Build history of the part. All positions in model axes, mm. A direction names the side the tool comes from. Give positions to 0.01 mm unless a question says otherwise; leave off trailing zeros. Loops run counter-clockwise (first coordinate to the right, second up) from the corner with the lowest first, then second, coordinate; pieces in that order, holes last. Notation, with made-up numbers: M 64,-6 L 122,-6 A29 ccw 122,22 Z; hole C -26,81.5 d2. An arc over 180 degrees is marked long. Answer in a Markdown table with one row per item. Add a question column.
```python
from build123d import *

# Parameters (mm, degrees)
SKETCH9_W           = 299
SKETCH9_H           = 464
SKETCH9_R           = 12.5
SKETCH9_R_2         = 10.287
SKETCH9_W_2         = 187.325
SKETCH9_H_2         = 265.1125
BOSS_EXTRUDE7_DEPTH = 3.175
FILLET4_R           = 10
FILLET5_R           = 12.7
SKETCH10_R          = 3
CUT_EXTRUDE1_DEPTH  = 3.175


with BuildPart() as part:
    # Sketch9 → Boss-Extrude7 (new body)
    with BuildSketch(Plane(origin=(0, 0, 0), x_dir=(1, 0, 0), z_dir=(0, 1, 0))):
        with Locations((0, 232)):
            Rectangle(SKETCH9_W, SKETCH9_H)
        with Locations(Location((-98.7, 63.5, 0), (0, 0, 270))):
            Circle(SKETCH9_R, mode=Mode.SUBTRACT)
        with Locations(Location((111.4, 76.2, 0), (0, 0, 270))):
            Circle(SKETCH9_R_2, mode=Mode.SUBTRACT)
        with Locations(Location((111.4, 38.1, 0), (0, 0, 270))):
            Circle(SKETCH9_R_2, mode=Mode.SUBTRACT)
        with Locations(Location((73.3, 76.2, 0), (0, 0, 270))):
            Circle(SKETCH9_R_2, mode=Mode.SUBTRACT)
        with Locations(Location((73.3, 38.1, 0), (0, 0, 270))):
            Circle(SKETCH9_R_2, mode=Mode.SUBTRACT)
        with Locations((9.5, 252)):
            Rectangle(SKETCH9_W_2, SKETCH9_H_2, mode=Mode.SUBTRACT)
        with BuildLine():
            Line((6.870225615, 415.1), (-6.870225615, 415.1))
            ThreePointArc((-6.870225615, 415.1), (0, 438.7), (6.870225615, 415.1))
        make_face(mode=Mode.SUBTRACT)
    extrude(amount=BOSS_EXTRUDE7_DEPTH)

    # Fillet4
    fillet4_edges = [part.edges().sort_by_distance(p)[0] for p in [
        (-149.5, 1.5875, -464),
        (149.5, 1.5875, -464),
        (149.5, 1.5875, 0),
        (-149.5, 1.5875, 0),
    ]]
    fillet(fillet4_edges, radius=FILLET4_R)

    # Fillet5
    fillet5_edges = [part.edges().sort_by_distance(p)[0] for p in [
        (103.1625, 1.5875, -119.44375),
        (103.1625, 1.5875, -384.55625),
        (-84.1625, 1.5875, -384.55625),
        (-84.1625, 1.5875, -119.44375),
    ]]
    fillet(fillet5_edges, radius=FILLET5_R)

    # Sketch10 → Cut-Extrude1 (cut)
    with BuildSketch(Plane(origin=(0, 3.175, 0), x_dir=(1, 0, 0), z_dir=(0, 1, 0))):
        with Locations(Location((-138.5, 11, 0), (0, 0, 270))):
            Circle(SKETCH10_R)
        with Locations(Location((-46.166666667, 11, 0), (0, 0, 270))):
            Circle(SKETCH10_R)
        with Locations(Location((46.166666667, 11, 0), (0, 0, 270))):
            Circle(SKETCH10_R)
        with Locations(Location((138.5, 11, 0), (0, 0, 270))):
            Circle(SKETCH10_R)
        with Locations(Location((-138.5, 84.666666667, 0), (0, 0, 270))):
            Circle(SKETCH10_R)
        with Locations(Location((-138.5, 158.333333333, 0), (0, 0, 270))):
            Circle(SKETCH10_R)
        with Locations(Location((-138.5, 232, 0), (0, 0, 270))):
            Circle(SKETCH10_R)
        with Locations(Location((-138.5, 305.666666667, 0), (0, 0, 270))):
            Circle(SKETCH10_R)
        with Locations(Location((-138.5, 379.333333333, 0), (0, 0, 270))):
            Circle(SKETCH10_R)
        with Locations(Location((-138.5, 453, 0), (0, 0, 270))):
            Circle(SKETCH10_R)
        with Locations(Location((138.5, 84.666666667, 0), (0, 0, 270))):
            Circle(SKETCH10_R)
        with Locations(Location((138.5, 158.333333333, 0), (0, 0, 270))):
            Circle(SKETCH10_R)
        with Locations(Location((138.5, 232, 0), (0, 0, 270))):
            Circle(SKETCH10_R)
        with Locations(Location((138.5, 305.666666667, 0), (0, 0, 270))):
            Circle(SKETCH10_R)
        with Locations(Location((138.5, 379.333333333, 0), (0, 0, 270))):
            Circle(SKETCH10_R)
        with Locations(Location((-46.166666667, 453, 0), (0, 0, 270))):
            Circle(SKETCH10_R)
        with Locations(Location((46.166666667, 453, 0), (0, 0, 270))):
            Circle(SKETCH10_R)
        with Locations(Location((138.5, 453, 0), (0, 0, 270))):
            Circle(SKETCH10_R)
    extrude(amount=-CUT_EXTRUDE1_DEPTH, mode=Mode.SUBTRACT)


solid = part.part
```
(1) Slice it at B-B, the plane z = -364.5. Give the cut face in (x, y) (1 decimal), then the cut area to 3 significant figures.
(2) Slice it at A-A, the plane x = -20. Give the cut face in (y, z) (3 decimals), then the cut area to 3 significant figures.
(3) Pin check, flat tip, straight feed: pin 1 (5.5 mm diameter, centred on x = 138.5, z = -84.67, fed in from +Y). Stop position of the tip, or through.
(4) Slice it at D-D, the plane x = 67.5. Give the cut face in (y, z) (3 decimals), then the cut area to 3 significant figures.
(5) Tool access for faces 1 (the cylindrical face through (-146.65, 1.61, -3.01)), 2 (the cylindrical face through (99.54, 1.61, -380.74)): list every direction of +Z, -Z, +X, -X, +Y, -Y with a clear straight run to the whole face (end or side of a thin tool).
(6) Slice it at C-C, the plane z = -38.1. Give the cut face in (x, y) (3 decimals).
(7) Pull direction Z, two halves, no side cores. Call faces 3 (the cylindrical face through (146.49, 1.61, -2.85)), 4 (the cylindrical face through (-146.65, 1.61, -460.99)), 5 (the cylindrical face through (-80.343, 1.61, -123.065)), 6 (the flat face through (-102, 0, -235)): +Z half, -Z half, draft (parallel to the pull), parting line (faces both ways), or undercut.
(8) Wall check: line 1 (X direction, y = 1.95, z = -453); line 2 (X direction, y = 2.25, z = -237); line 3 (Z direction, x = -10, y = 0.5). Give the ranges that are in metal, low to high.
Solution:
| question | item | result |
|---|---|---|
| 1 | outline | M -149.5,0 L -84.2,0 L -84.2,3.2 L -149.5,3.2 Z; M 103.2,0 L 149.5,0 L 149.5,3.2 L 103.2,3.2 Z |
| 1 | area | 355 mm^2 |
| 2 | outline | M 0,-464 L 3.175,-464 L 3.175,-384.556 L 0,-384.556 Z; M 0,-119.444 L 3.175,-119.444 L 3.175,0 L 0,0 Z |
| 2 | area | 631 mm^2 |
| 3 | pin 1 | through |
| 4 | outline | M 0,-464 L 3.175,-464 L 3.175,-384.556 L 0,-384.556 Z; M 0,-119.444 L 3.175,-119.444 L 3.175,-84.696 L 0,-84.696 Z; M 0,-67.704 L 3.175,-67.704 L 3.175,-46.596 L 0,-46.596 Z; M 0,-29.604 L 3.175,-29.604 L 3.175,0 L 0,0 Z |
| 4 | area | 524 mm^2 |
| 5 | face 1 | +Z, -X, +Y, -Y |
| 5 | face 2 | +Y, -Y |
| 6 | outline | M -149.5,0 L 63.013,0 L 63.013,3.175 L -149.5,3.175 Z; M 83.587,0 L 101.113,0 L 101.113,3.175 L 83.587,3.175 Z; M 121.687,0 L 149.5,0 L 149.5,3.175 L 121.687,3.175 Z |
| 7 | face 3 | +Z half |
| 7 | face 4 | -Z half |
| 7 | face 5 | undercut |
| 7 | face 6 | draft |
| 8 | line 1 | -149.5 to -141.5, -135.5 to -49.17, -43.17 to 43.17, 49.17 to 135.5, 141.5 to 149.5 |
| 8 | line 2 | -149.5 to -84.16, 103.16 to 149.5 |
| 8 | line 3 | -464 to -433.89, -417.91 to -384.56, -119.44 to 0 |
